Design review of the part built by this model. Coordinates are the model's own, in mm. A direction names the side the tool comes from. Coordinates: 2 decimals unless noted, no trailing zeros. Loops run counter-clockwise (first coordinate to the right, second up) from the corner with the lowest first, then second, coordinate; pieces in that order, holes last. Notation, with made-up numbers: (75, 9.25) - (86, 9.25) arc R13 cw to (86, 13.25) - close; hole circle Ø10 at (-20.75, -28). An arc over 180 degrees is marked (long way). Answer in a Markdown table with one row per item. Add a question column.
(1) To check wall thickness, follow L1, parallel to X at y = -2.75, z = 420; L2, parallel to Z at x = 0, y = -8.55; L3, parallel to X at y = 6.25, z = 290.5. State the ranges of each line that lie inside material, in increasing order. Write a range as [from, to].
(2) We need section C-C, the plane x = -28. Write out the cut boundary in (y, z).
(3) The part is to be moulded in two halves that separate along Y. For faces 3 (the face through (-60, 0, 308)), 4 (the face through (1, -9, 308)), 5 (the face through (0, -7.2, 308)), say which applies: released by +Y, released by -Y, zero draft, split by the parting line, or undercut.
(4) We need section A-A, the plane y = -3.75. Write out the cut boundary in (x, z).
(5) For faces 1 (the face through (-4, -8, 625)), 2 (the face through (35, -7.2, 308)), list the 3-axis set-ups (+Z, -Z, +X, -X, +Y, -Y) from which the entire face can be reached by the end or side of a thin tool; tool diameter is ignored.
(6) We need section B-B, the plane z = 47.5. Write out the cut boundary in (x, y).
(7) Clearance check with a flat-ended pin moving along its axis: pin 1 (3 mm diameter, centred on x = 0, z = 603, fed in from -Y). State where the tip first meets the part, or that it passes through.
from build123d import *

# Parameters (mm, degrees)
SKETCH1_W                  = 45
SKETCH1_H                  = 14.4
BOSS_EXTRUDE1_DEPTH        = 625
F_5_2_5_2_DIAMETER_HOLE1_D = 5.2


with BuildPart() as part:
    # Sketch1 → Boss-Extrude1 (new body)
    with BuildSketch(Plane.XY):
        Polygon((-10.5, 5.2), (-10.5, -7.2), (10.5, -7.2), (10.5, 5.2), (5.5, 5.2), (5.5, 9), (60, 9), (60, -9), (-60, -9), (-60, 9), (-5.5, 9), (-5.5, 5.2), align=None)
        with Locations((-35.7, 0)):
            Rectangle(SKETCH1_W, SKETCH1_H, mode=Mode.SUBTRACT)
        with Locations((35.7, 0)):
            Rectangle(SKETCH1_W, SKETCH1_H, mode=Mode.SUBTRACT)
    extrude(amount=BOSS_EXTRUDE1_DEPTH)

    # Ø5.2 (5.2) Diameter Hole1 (through all)
    with Locations(Plane(origin=(0, -9, 0), x_dir=(-1, 0, 0), z_dir=(0, -1, 0))):
        with Locations((0, -22), (0, -603)):
            Hole(F_5_2_5_2_DIAMETER_HOLE1_D / 2)


solid = part.part
Responses:
| question | item | result |
|---|---|---|
| 1 | L1 | x = [-60, -58.2], [-13.2, -10.5], [10.5, 13.2], [58.2, 60] |
| 1 | L2 | z = [0, 19.4], [24.6, 600.4], [605.6, 625] |
| 1 | L3 | x = [-60, -58.2], [-13.2, -5.5], [5.5, 13.2], [58.2, 60] |
| 2 | outline | (-9, 0) - (-7.2, 0) - (-7.2, 625) - (-9, 625) - close; (7.2, 0) - (9, 0) - (9, 625) - (7.2, 625) - close |
| 3 | face 3 | zero draft |
| 3 | face 4 | released by -Y |
| 3 | face 5 | undercut |
| 4 | outline | (-60, 0) - (-58.2, 0) - (-58.2, 625) - (-60, 625) - close; (-13.2, 0) - (-10.5, 0) - (-10.5, 625) - (-13.2, 625) - close; (10.5, 0) - (13.2, 0) - (13.2, 625) - (10.5, 625) - close; (58.2, 0) - (60, 0) - (60, 625) - (58.2, 625) - close |
| 5 | face 1 | +Z, +X, -X, +Y, -Y |
| 5 | face 2 | +Z, -Z |
| 6 | outline | (-60, -9) - (60, -9) - (60, 9) - (5.5, 9) - (5.5, 5.2) - (10.5, 5.2) - (10.5, -7.2) - (-10.5, -7.2) - (-10.5, 5.2) - (-5.5, 5.2) - (-5.5, 9) - (-60, 9) - close; hole (-58.2, -7.2) - (-13.2, -7.2) - (-13.2, 7.2) - (-58.2, 7.2) - close; hole (13.2, -7.2) - (58.2, -7.2) - (58.2, 7.2) - (13.2, 7.2) - close |
| 7 | pin 1 | passes through |
